Part model, mm, in its own coordinate system. Face numbers are marked on the shaded views. A direction names the side the tool comes from. Give positions to 0.01 mm unless a question says otherwise; leave off trailing zeros. Order: outer loops, then holes, each group sorted by start corner. A loop starts at its lowest first (then second) coordinate and runs counter-clockwise, first axis right, second up. Notation, with made-up numbers: (-1.75, 23) -> (53.25, 23) arc R13 ccw to (53.25, 32) -> close; hole circle Ø9 at (75, 16.5). An arc over 180 degrees is marked (long way). Write item = value, one per line. Start each with the question number.
Item 1: Drill centre lines: line 1 along Y through (x, z) = (75, 2.9); line 2 along Y through (x, z) = (95, 12.75); line 3 along Y through (x, z) = (12.5, 13.75). Where is each one in solid material? Low to high.
Item 2: Flat gauge pins, fed straight in: P1, Ø1.5, axis at x = 144, z = 2, coming from the -Y side; P2, Ø1.5, axis at x = 145.5, y = 5.5, coming from the -Z side. Where does each tip first touch, or does it go through?
Item 3: Pull direction X, two halves, no side cores. Call the marked faces 3, 4, 5 and 6: +X half, -X half, draft (parallel to the pull), parting line (faces both ways), or undercut.
Item 4: Tool access for the marked faces 1 and 2: list every direction of +Z, -Z, +X, -X, +Y, -Y with a clear straight run to the whole face (end or side of a thin tool).
Item 5: Band-saw the part on A-A on y = 50.5. Write the cut outline in (x, z).
Item 6: Band-saw the part on B-B on x = 75. Write the cut outline in (y, z).
Item 7: Band-saw the part on C-C on x = 136. Write the cut outline in (y, z).
Autodesk Inventor part; units mm, degrees
ref_plane "YZ Plane" through (0, 0, 0) normal (1, 0, 0) x (0, 1, 0)
ref_plane "XZ Plane" through (0, 0, 0) normal (0, 1, 0) x (-1, 0, 0)
ref_plane "XY Plane" through (0, 0, 0) normal (0, 0, 1) x (1, 0, 0)
sketch "Sketch4" plane through (0, 0, 0) normal (0, 0, 1) x (1, 0, 0)
  line L0 (0, 0) -> (150, 0)
  line L1 (150, 0) -> (150, 150)
  line L2 (150, 150) -> (0, 150)
  line L3 (0, 150) -> (0, 0)
  dimension "d34" = 150
  dimension "d35" = 150
extrude "Extrusion4" add sketch "Sketch4" along normal blind 10
sketch "Sketch5" plane through (0, 0, 10) normal (0, 0, 1) x (1, 0, 0)
  line L0 (10, 10) -> (140, 10)
  line L1 (140, 10) -> (140, 140)
  line L2 (140, 140) -> (10, 140)
  line L3 (10, 140) -> (10, 10)
  point P0 (0, 0)
  dimension "d38" = 130
  dimension "d39" = 130
extrude "Extrusion5" cut sketch "Sketch5" against normal blind 2
sketch "Sketch6" plane through (0, 0, 0) normal (0, 0, -1) x (-1, 0, 0)
  circle A0 centre (-75, 75) radius 14.25
  circle A1 centre (-75, 75) radius 17.15
  line L0 (-147.5, 2.5) -> (-142.5, 2.5)
  line L1 (-142.5, 2.5) -> (-142.5, 7.5)
  line L2 (-142.5, 7.5) -> (-147.5, 7.5)
  line L3 (-147.5, 7.5) -> (-147.5, 2.5)
  line L4 (-2.5, 2.5) -> (-7.5, 2.5)
  line L5 (-7.5, 2.5) -> (-7.5, 7.5)
  line L6 (-7.5, 7.5) -> (-2.5, 7.5)
  line L7 (-2.5, 7.5) -> (-2.5, 2.5)
  line L8 (-147.5, 147.5) -> (-142.5, 147.5)
  line L9 (-142.5, 147.5) -> (-142.5, 142.5)
  line L10 (-142.5, 142.5) -> (-147.5, 142.5)
  line L11 (-147.5, 142.5) -> (-147.5, 147.5)
  line L12 (-2.5, 147.5) -> (-7.5, 147.5)
  line L13 (-7.5, 147.5) -> (-7.5, 142.5)
  line L14 (-7.5, 142.5) -> (-2.5, 142.5)
  line L15 (-2.5, 142.5) -> (-2.5, 147.5)
  point P0 (0, 0)
  dimension "d42" = 28.5
  dimension "d43" = 34.3
  dimension "d46" = 5
  dimension "d47" = 5
  dimension "d48" = 5
  dimension "d49" = 5
  dimension "d50" = 5
  dimension "d51" = 5
  dimension "d52" = 5
  dimension "d53" = 5
extrude "Extrusion7" cut sketch "Sketch6" against normal blind 5
sketch "Sketch7" plane through (0, 0, 8) normal (0, 0, 1) x (1, 0, 0)
  line L0 (47.5, 102.5) -> (102.5, 102.5)
  line L1 (102.5, 102.5) -> (102.5, 47.5)
  line L2 (102.5, 47.5) -> (47.5, 47.5)
  line L3 (47.5, 47.5) -> (47.5, 102.5)
  point P0 (0, 0)
  dimension "d58" = 55
  dimension "d59" = 55
extrude "Extrusion8" cut sketch "Sketch7" against normal blind 2
sketch "Sketch9" plane through (0, 0, 6) normal (0, 0, 1) x (1, 0, 0)
  line L0 (47.5, 47.5) -> (47.5, 102.5)
  line L1 (47.5, 47.5) -> (102.5, 47.5)
  line L2 (102.5, 47.5) -> (102.5, 102.5)
  line L3 (102.5, 102.5) -> (47.5, 102.5)
  line L4 (47.5, 102.5) -> (47.5, 47.5)
  point P0 (0, 0)
  dimension "d68" = 55
  dimension "d69" = 55
extrude "Extrusion10" add sketch "Sketch9" along normal blind 2
sketch "Sketch10" plane through (0, 0, 8) normal (0, 0, 1) x (1, 0, 0)
  line L0 (37.5, 37.5) -> (112.5, 37.5)
  line L1 (112.5, 37.5) -> (112.5, 112.5)
  line L2 (37.5, 37.5) -> (112.5, 37.5)
  line L3 (112.5, 37.5) -> (112.5, 112.5)
  line L4 (112.5, 112.5) -> (37.5, 112.5)
  line L5 (37.5, 112.5) -> (37.5, 37.5)
  point P0 (0, 0)
  dimension "d72" = 75
  dimension "d73" = 75
extrude "Extrusion11" add sketch "Sketch10" along normal blind 5
sketch "Sketch11" plane through (0, 0, 13) normal (0, 0, 1) x (1, 0, 0)
  line L0 (47.5, 47.5) -> (102.5, 47.5)
  line L1 (102.5, 47.5) -> (102.5, 102.5)
  line L2 (102.5, 102.5) -> (47.5, 102.5)
  line L3 (47.5, 102.5) -> (47.5, 47.5)
  point P0 (0, 0)
  dimension "d76" = 55
  dimension "d77" = 55
extrude "Extrusion12" cut sketch "Sketch11" against normal blind 2
sketch "Sketch12" plane through (0, 0, 11) normal (0, 0, 1) x (1, 0, 0)
  circle A0 centre (75, 75) radius 14.35
  circle A1 centre (75, 75) radius 17.15
  point P0 (0, 0)
sketch "Sketch13" plane through (0, 0, 8) normal (0, 0, 1) x (1, 0, 0)
  line L0 (140, 140) -> (140, 10)
  line L1 (10, 140) -> (140, 140)
  line L2 (140, 140) -> (140, 10)
  line L3 (140, 10) -> (10, 10)
  line L4 (10, 10) -> (10, 140)
  line L5 (37.5, 37.5) -> (37.5, 112.5)
  line L6 (112.5, 112.5) -> (112.5, 37.5)
  line L7 (37.5, 112.5) -> (112.5, 112.5)
  line L8 (112.5, 112.5) -> (112.5, 37.5)
  line L9 (112.5, 37.5) -> (37.5, 37.5)
  line L10 (37.5, 37.5) -> (37.5, 112.5)
  point P0 (0, 0)
extrude "Extrusion13" add sketch "Sketch13" along normal blind 5
sketch "Sketch15" plane through (0, 0, 10) normal (0, 0, 1) x (1, 0, 0)
  line L0 (0, 0) -> (150, 0)
  line L1 (150, 0) -> (150, 150)
  line L2 (150, 150) -> (0, 150)
  line L3 (0, 150) -> (0, 0)
  line L4 (10, 140) -> (10, 10)
  line L5 (10, 140) -> (140, 140)
  line L6 (140, 140) -> (140, 10)
  line L7 (140, 10) -> (10, 10)
  line L8 (10, 10) -> (10, 140)
  dimension "d86" = 150
  dimension "d87" = 150
  dimension "d88" = 130
  dimension "d89" = 130
extrude "Extrusion14" add sketch "Sketch15" along normal blind 5
properties part number "Elbow_Both_Marker_TestFit_V2"
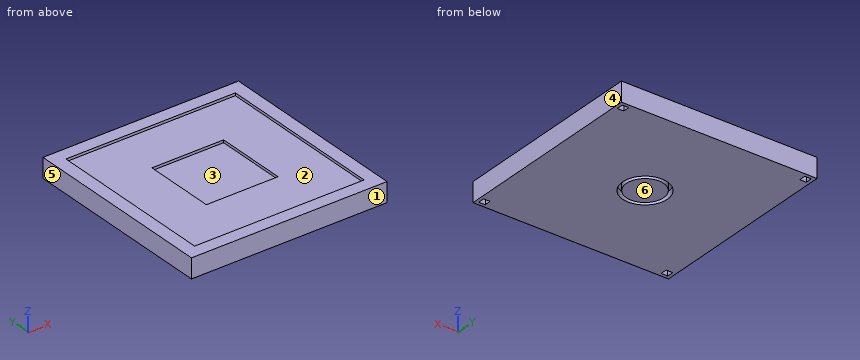
Values found:
q1.line_1 = 0 to 57.85, 60.75 to 89.25, 92.15 to 150
q1.line_2 = 0 to 47.5, 102.5 to 150
q1.line_3 = 0 to 10, 140 to 150
q2.P1 = 0
q2.P2 = 5
q3.face_3 = undercut
q3.face_4 = +X half
q3.face_5 = -X half
q3.face_6 = draft
q4.face_1 = +Z, -Z, +X, -X, -Y
q4.face_2 = +Z
q5.outline = (0, 0) -> (150, 0) -> (150, 15) -> (140, 15) -> (140, 13) -> (102.5, 13) -> (102.5, 11) -> (47.5, 11) -> (47.5, 13) -> (10, 13) -> (10, 15) -> (0, 15) -> close
q6.outline = (0, 0) -> (57.85, 0) -> (57.85, 5) -> (60.75, 5) -> (60.75, 0) -> (89.25, 0) -> (89.25, 5) -> (92.15, 5) -> (92.15, 0) -> (150, 0) -> (150, 15) -> (140, 15) -> (140, 13) -> (102.5, 13) -> (102.5, 11) -> (47.5, 11) -> (47.5, 13) -> (10, 13) -> (10, 15) -> (0, 15) -> close
q7.outline = (0, 0) -> (150, 0) -> (150, 15) -> (140, 15) -> (140, 13) -> (10, 13) -> (10, 15) -> (0, 15) -> close
